Answer from the drawing. Dimensions are ordinates in mm from the lowest x, y and z of the part. A direction names the side the tool comes from. Round coordinates to 2 decimals unless told otherwise and drop trailing zeros. Loops run counter-clockwise (first coordinate to the right, second up) from the corner with the lowest first, then second, coordinate; pieces in that order, holes last. Notation, with made-up numbers: (74.5, 20.5) - (88.5, 20.5) arc R12 ccw to (88.5, 24.5) - close; hole circle Ø8 at (8.5, 85). An arc over 180 degrees is marked (long way). Return JSON: item names as keys, results as strings.
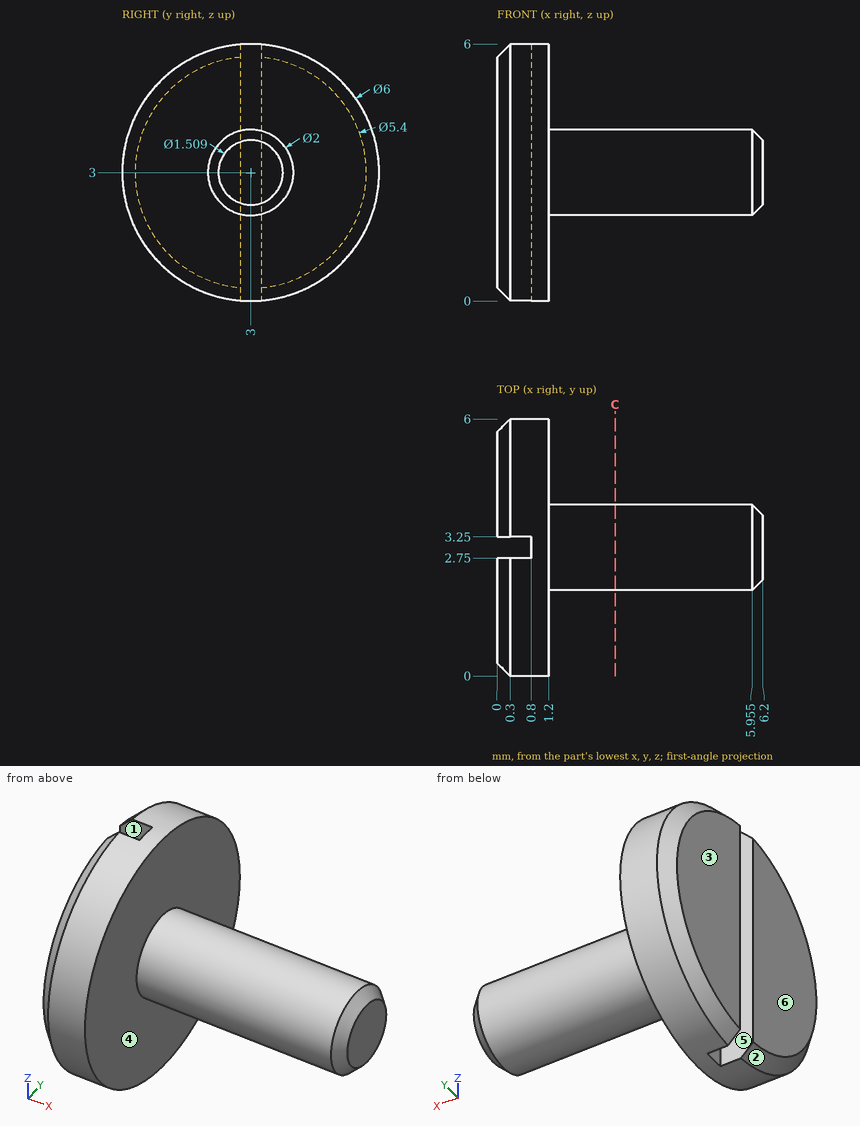
1) Determine the mould class of the marked faces 1, 2 and 3 for opening direction Y: pulls with the +Y half, pulls with the -Y half, needs draft (parallel to the pull), parting line crosses it, or undercut.
Verdict:
{"face 1": "undercut", "face 2": "pulls with the -Y half", "face 3": "needs draft"}
2) Section C-C (x = 2.75) is taken. Give the vertices of the cut face in (y, z).
Verdict:
{"outline": "circle Ø2 at (3, 3)"}
3) A tool of negligible diameter and unlimited length cuts with its end or side. For the marked faces 4, 5 and 6, from which of +Z, -Z, +X, -X, +Y, -Y can it reach the whole face along a straight path? Write none if from no direction.
Verdict:
{"face 4": "+X", "face 5": "+Z, -Z, -X", "face 6": "+Z, -Z, -X, +Y, -Y"}
4) Flat-ended cylindrical pins translate along their axes: pin 1 (3 mm diameter, centred on x = 5, z = 5, fed in from -Y) (1 decimal); pin 2 (2 mm diameter, centred on x = 4, z = 4.5, fed in from +Y) (1 decimal); pin 3 (0.9 mm diameter, centred on x = 0.5, z = 4.5, fed in from -Y). Find the tip coordinate at first contact, or state that the pin passes through.
Verdict:
{"pin 1": "stops at y = 2.1", "pin 2": "stops at y = 3.9", "pin 3": "stops at y = 0.19"}
5) Find the intervals of material crossed by L1, parallel to X at y = 3.75, z = 1; L2, parallel to Y at x = 2, z = 3.25; L3, parallel to Z at x = 1, y = 5 (1 decimal), in increasing order.
Verdict:
{"L1": "x = 0 to 1.2", "L2": "y = 2.03 to 3.97", "L3": "z = 0.8 to 5.2"}
